Part print with two shaded views. Sizes in mm from the minimum x, y, z corner. Coordinates: 2 decimals unless noted, no trailing zeros. Loops run counter-clockwise (first coordinate to the right, second up) from the corner with the lowest first, then second, coordinate; pieces in that order, holes last.
(1) Slice it at A-A (z = 15). Give the cut face in (x, y), and give its area (3 significant figures).
(2) Wall check: L1, parallel to Z at x = 185, y = 6; L2, parallel to X at y = 6, z = 189. Give the ranges that are in metal, low to high.
(3) Flat gauge pin, fed straight in: P1, Ø2.5, axis at x = 121.21, z = 78.79, coming from the +Y side. Where does the tip first touch, or does it go through?
(4) Slice it at B-B (x = 15). Give the cut face in (y, z).
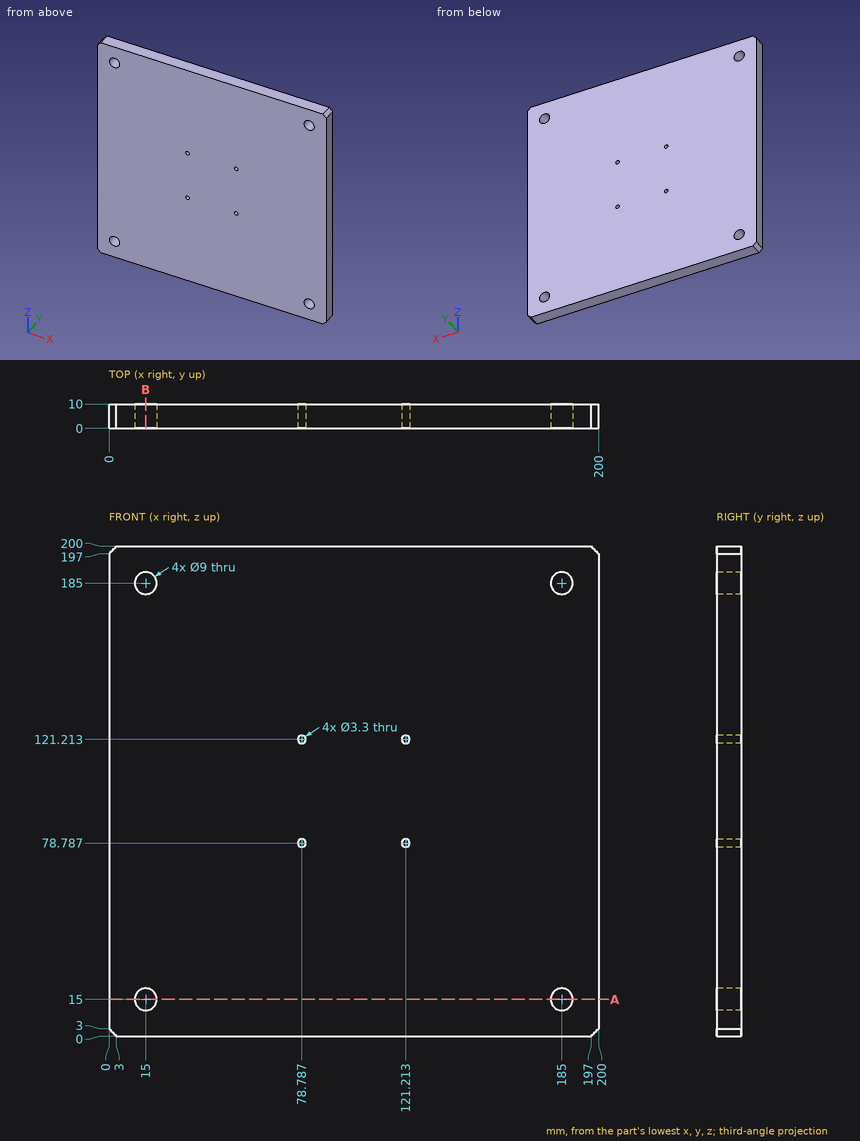
Response values:
1. outline: (0, 0) - (10.5, 0) - (10.5, 10) - (0, 10) - close; (19.5, 0) - (180.5, 0) - (180.5, 10) - (19.5, 10) - close; (189.5, 0) - (200, 0) - (200, 10) - (189.5, 10) - close
1. area: 1,820 mm2
2. L1: z = 0 to 10.5, 19.5 to 180.5, 189.5 to 200
2. L2: x = 0 to 12.94, 17.06 to 182.94, 187.06 to 200
3. P1: passes through
4. outline: (0, 0) - (10, 0) - (10, 10.5) - (0, 10.5) - close; (0, 19.5) - (10, 19.5) - (10, 180.5) - (0, 180.5) - close; (0, 189.5) - (10, 189.5) - (10, 200) - (0, 200) - close
